Autodesk Inventor part; units mm, degrees
ref_plane "YZ Plane" through (0, 0, 0) normal (1, 0, 0) x (0, 1, 0)
ref_plane "XZ Plane" through (0, 0, 0) normal (0, 1, 0) x (-1, 0, 0)
ref_plane "XY Plane" through (0, 0, 0) normal (0, 0, 1) x (1, 0, 0)
sketch "Sketch1" plane through (0, 0, 0) normal (0, 0, 1) x (1, 0, 0)
  line L0 (0, 0) -> (-330.2, 0)
  line L1 (-330.2, 0) -> (-330.2, 50.8)
  line L2 (-330.2, 50.8) -> (0, 50.8)
  line L3 (0, 50.8) -> (0, 0)
  circle A0 centre (-12.7, 38.1) radius 3.1
  circle A1 centre (-12.7, 12.7) radius 3.1
  circle A2 centre (-317.5, 38.1) radius 3.1
  circle A3 centre (-317.5, 12.7) radius 3.1
  circle A4 centre (-285.75, 25.4) radius 3
  circle A5 centre (-44.45, 25.4) radius 3
  dimension "d0" = 330.2
  dimension "d1" = 50.8
  dimension "d2" = 6.2
  dimension "d3" = 6.2
  dimension "d4" = 6.2
  dimension "d5" = 6.2
  dimension "d6" = 12.7
  dimension "d7" = 12.7
  dimension "d8" = 25.4
  dimension "d9" = 12.7
  dimension "d10" = 12.7
  dimension "d11" = 12.7
  dimension "d12" = 25.4
  dimension "d13" = 12.7
  dimension "d16" = 6
  dimension "d17" = 44.45
  dimension "d18" = 6
  dimension "d19" = 44.45
extrude "Extrusion1" add sketch "Sketch1" along normal blind 6.35 contours L0 L1 L2 L3 | A4 | A5
sketch "Sketch2" plane through (0, 0, 6.35) normal (0, 0, 1) x (1, 0, 0)
  circle A0 centre (-44.45, 25.4) radius 3
  circle A1 centre (-285.75, 25.4) radius 3
  line L0 (0, 0) -> (0, 50.8)
  line L1 (-330.2, 50.8) -> (-330.2, 0)
  dimension "d20" = 6
  dimension "d21" = 6
  dimension "d22" = 44.45
  dimension "d23" = 44.45
extrude "Extrusion2" cut sketch "Sketch2" against normal blind 6.35
properties part number "outbrace" material "Aluminum 6061"
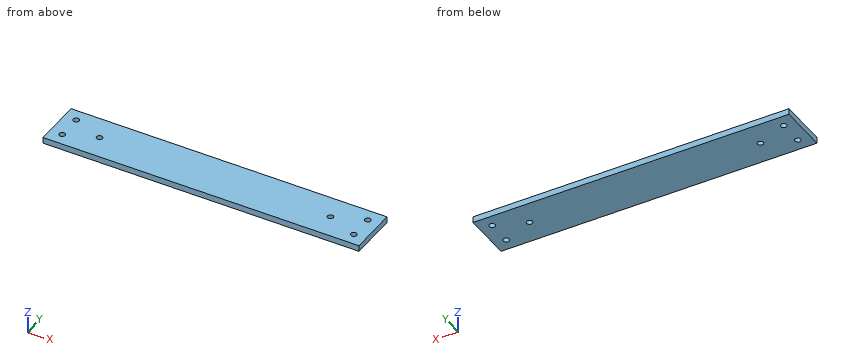
Here's how the part is built. I have some questions about the finished solid (model axes, mm). Round coordinates to 2 decimals unless told otherwise and drop trailing zeros. Loops run counter-clockwise (first coordinate to the right, second up) from the corner with the lowest first, then second, coordinate; pieces in that order, holes last. Notation, with made-up numbers: (-35.5, -38.75) -> (2.5, -38.75) arc R16 ccw to (2.5, -19.75) -> close; hole circle Ø10 at (-3.5, 85.5). An arc over 180 degrees is marked (long way). Answer as CSV lines item,"result". Start each with the question number.
1. Imagine slicing it at A-A on x = -317.5. Write out the boundary of the cut face in (y, z), plus the area to 3 significant figures.
2. I'm going to push a flat-ended pin straight in: P1, Ø3.5, axis at x = -44.45, y = 25.4, coming from the +Z side. Where does the tip first touch, or does it pass through?
3. Imagine slicing it at B-B on y = 25.4. Write out the boundary of the cut face in (x, z), plus the area to 3 significant figures.
4. I need wall thicknesses on probe 1 along Y at (x, z) = (-12.7, 4.5); probe 2 along Y at (x, z) = (-285.75, 3); probe 3 along X at (y, z) = (36.5, 2.5). Which ranges of each line are inside material? Lowest first, please. Write a range as from..to.
Solution:
1,outline,"(0, 0) -> (9.6, 0) -> (9.6, 6.35) -> (0, 6.35) -> close; (15.8, 0) -> (35, 0) -> (35, 6.35) -> (15.8, 6.35) -> close; (41.2, 0) -> (50.8, 0) -> (50.8, 6.35) -> (41.2, 6.35) -> close"
1,area,"244 mm²"
2,P1,"through"
3,outline,"(-330.2, 0) -> (-288.75, 0) -> (-288.75, 6.35) -> (-330.2, 6.35) -> close; (-282.75, 0) -> (-47.45, 0) -> (-47.45, 6.35) -> (-282.75, 6.35) -> close; (-41.45, 0) -> (0, 0) -> (0, 6.35) -> (-41.45, 6.35) -> close"
3,area,"2,020 mm²"
4,probe 1,"0..9.6, 15.8..35, 41.2..50.8"
4,probe 2,"0..22.4, 28.4..50.8"
4,probe 3,"-330.2..-320.16, -314.84..-15.36, -10.04..0"
